Source: CAD feature listing. Evaluate the final solid. Frame: model axes, mm. Coordinates: 2 decimals unless noted, no trailing zeros. Write each loop counter-clockwise with the first axis right and the second up, starting at its lowest first coordinate (ties: lowest second). Pieces come first, ordered by that corner, then holes. Notation, with made-up numbers: M 21.25,71.5 L 79.25,71.5 A14 cw 79.25,75.5 Z; hole C 68,3.25 d1. An arc over 180 degrees is marked long. Answer as CSV lines item,"result". Start each with the question number.
1. Section B-B on y = 18.5. Return the cut outline in (x, z).
2. Line query: probe 1 along Y at (x, z) = (-3, 23.5); probe 2 along Y at (x, z) = (13, 15.5); probe 3 along X at (y, z) = (-6.5, 2.5). Output: solid intervals per line, ascending. Write a range as [from, to].
3. Contact query for flat-ended pins moving along their axis: pin 1 Ø1.5 at (y, z) = (12.5, 12.5) entering from +X; pin 2 Ø4 at (y, z) = (13.5, 22) entering from +X; pin 3 Ø1 at (x, y) = (-14, -13) entering from -Z; pin 4 Ø8 at (y, z) = (-10.5, 9) entering from +X. Output: stop coordinate, or through.
4. Section C-C on x = -14.5. Return the cut outline in (y, z).
5. Section A-A on z = 8. Return the cut outline in (x, y).
```python
from build123d import *

# Parameters (mm, degrees)
F1_DEPTH = 25


with BuildPart() as f1:
    # F0 (on Top) → F1 (new body)
    with BuildSketch(Plane.XY):
        Polygon((-17.67767, 17.67767), (-18.141327, 17.67767), (-20.478801, 14.339411), (0, 0), align=None)
        Polygon((16.557725, 23.646883), (-12.199938, 26.162852), (-18.141327, 17.67767), (-17.67767, 17.67767), (0, 0), (-20.478801, 14.339411), (-28.757664, 2.51597), (-16.557725, -23.646883), (12.199938, -26.162852), (28.757664, -2.51597), align=None)
    extrude(amount=F1_DEPTH)


solid = f1.part
```
Values:
1,outline,"M -17.57,0 L 18.96,0 L 18.96,25 L -17.57,25 Z"
2,probe 1,"[-24.83, 25.36]"
2,probe 2,"[-25.02, 23.96]"
2,probe 3,"[-24.55, 25.97]"
3,pin 1,"x = 22.11"
3,pin 2,"x = 22.22"
3,pin 3,"z = 0"
3,pin 4,"x = 25.97"
4,outline,"M -23.83,0 L 22.88,0 L 22.88,25 L -23.83,25 Z"
5,outline,"M -28.76,2.52 L -16.56,-23.65 L 12.2,-26.16 L 28.76,-2.52 L 16.56,23.65 L -12.2,26.16 Z"
